```python
from build123d import *

# Parameters (mm, degrees)
BOSS_EXTRUDE1_DEPTH = 9.652
SKETCH2_R           = 2.54
CUT_EXTRUDE1_DEPTH  = 5.08


with BuildPart() as part:
    # Sketch1 → Boss-Extrude1 (new body)
    with BuildSketch(Plane.XY):
        with BuildLine():
            Line((2476.991807356, 1418.793197854), (2476.991807356, 1431.493197854))
            Line((2476.991807356, 1431.493197854), (2512.043807356, 1431.493197854))
            Line((2512.043807356, 1431.493197854), (2512.043807356, 1417.89780113))
            Line((2512.043807356, 1417.89780113), (2504.92216143, 1417.89780113))
            ThreePointArc((2504.92216143, 1417.89780113), (2495.135108983, 1426.393265728), (2484.637572003, 1418.793197854))
            Line((2484.637572003, 1418.793197854), (2476.991807356, 1418.793197854))
        make_face()
    extrude(amount=BOSS_EXTRUDE1_DEPTH)

    # Sketch2 → Cut-Extrude1 (cut)
    with BuildSketch(Plane(origin=(0, 1431.493197854, 0), x_dir=(1, 0, 0), z_dir=(0, 1, 0))):
        with Locations(Location((2483.087807356, -4.826, 0), (0, 0, 270))):
            Circle(SKETCH2_R)
        with Locations(Location((2505.947807356, -4.826, 0), (0, 0, 90))):
            Circle(SKETCH2_R)
    extrude(amount=-CUT_EXTRUDE1_DEPTH, mode=Mode.SUBTRACT)


solid = part.part
```
Geometry: final body of the model. Coordinates: model frame, mm. A direction names the side the tool comes from. Give positions to 0.01 mm unless a question says otherwise; leave off trailing zeros. Loops run counter-clockwise (first coordinate to the right, second up) from the corner with the lowest first, then second, coordinate; pieces in that order, holes last. Notation, with made-up numbers: (55.25, 68.5) - (113.25, 68.5) arc R11 ccw to (113.25, 76.5) - close; hole circle Ø9 at (63.5, 23). An arc over 180 degrees is marked (long way). Answer as CSV lines item,"result". Start each with the question number.
(1) Section query B-B (z = 8.5). Output: boundary loops of the cut face in (x, y) (3 decimals), and give its area (3 significant figures).
(2) Section query C-C (y = 1423.75). Output: boundary loops of the cut face in (x, z), and give its area (3 significant figures).
(3) Section query A-A (y = 1420.5). Output: boundary loops of the cut face in (x, z), and give its area (3 significant figures).
(4) Section query D-D (y = 1429.5). Output: boundary loops of the cut face in (x, z).
(5) Pin query (flat end, axial travel): P1, Ø4.5, axis at x = 2483.09, z = 4.83, coming from the -Y side; P2, Ø2.5, axis at x = 2484, z = 4, coming from the +Y side; P3, Ø5, axis at x = 2487.5, z = 2, coming from the -Y side. Return the tip coordinate at first contact, or that it passes through.
(6) Reachability of faces 1 (the face through (2506, 1426.413, 5)), 2 (the face through (2495.331, 1426.383, 4.758)), 3 (the face through (2481, 1418.793, 5)) from +Z, -Z, +X, -X, +Y, -Y: full face, straight path, thin tool, end or side. Return the list, or none.
(7) Ray query, line 1 along X through (y, z) = (1430.5, 3.5); line 2 along Y through (x, z) = (2482.5, 8); line 3 along X through (y, z) = (1419.25, 5). Return the intervals inside material, ascending. Write a range as [from, to].
Worked answers:
1,outline,"(2476.992, 1418.793) - (2484.638, 1418.793) arc R10.425 cw to (2504.922, 1417.898) - (2512.044, 1417.898) - (2512.044, 1431.493) - (2476.992, 1431.493) - close"
1,area,"339 mm^2"
2,outline,"(2476.99, 0) - (2487.73, 0) - (2487.73, 9.65) - (2476.99, 9.65) - close; (2501.62, 0) - (2512.04, 0) - (2512.04, 9.65) - (2501.62, 9.65) - close"
2,area,"204 mm^2"
3,outline,"(2476.99, 0) - (2485.28, 0) - (2485.28, 9.65) - (2476.99, 9.65) - close; (2504.07, 0) - (2512.04, 0) - (2512.04, 9.65) - (2504.07, 9.65) - close"
3,area,"157 mm^2"
4,outline,"(2476.99, 0) - (2512.04, 0) - (2512.04, 9.65) - (2476.99, 9.65) - close; hole circle Ø5.08 at (2483.09, 4.83); hole circle Ø5.08 at (2505.95, 4.83)"
5,P1,"stops at y = 1418.79"
5,P2,"stops at y = 1426.41"
5,P3,"stops at y = 1419.86"
6,face 1,"+Y"
6,face 2,"+Z, -Z, -Y"
6,face 3,"+Z, -Z, -X, -Y"
7,line 1,"x = [2476.99, 2480.92], [2485.25, 2503.78], [2508.11, 2512.04]"
7,line 2,"y = [1418.79, 1431.49]"
7,line 3,"x = [2476.99, 2484.78], [2504.57, 2512.04]"
